Input: part model. Units: mm. Frame: model coordinates. A direction names the side the tool comes from. Give positions to 0.01 mm unless a question says otherwise; leave off trailing zeros. Order: outer loops, then holes, each group sorted by start corner. A loop starts at its lowest first (then second) coordinate and runs counter-clockwise, first axis right, second up. Notation, with made-up numbers: (-32.5, 17.5) - (-18.5, 17.5) arc R12 cw to (-18.5, 38.5) - close; hole circle Ø6 at (76, 39.25). An arc over 180 degrees is marked (long way). Answer in a Markdown table with one row per item. Add a question column.
from build123d import *

# Parameters (mm, degrees)
F1_DEPTH = 254
F2_R     = 1.98374
F3_R     = 3.69316
F4_R     = 1.35255
F5_DEPTH = 171.69384
F6_R     = 1.8288
F7_DEPTH = 1.70942
F8_R     = 0.762


with BuildPart() as f1:
    # F0 (on Top) → F1 (new body)
    with BuildSketch(Plane.XY):
        Polygon((0, -161.925), (0, 0), (-11.63066, 0), (-11.63066, -1.70942), (-1.70942, -1.70942), (-1.70942, -163.63442), (169.98442, -163.63442), (169.98442, -1.70942), (179.90566, -1.70942), (179.90566, 0), (168.275, 0), (168.275, -161.925), align=None)
    extrude(amount=F1_DEPTH)

    # F2
    f2_edges = [f1.edges().sort_by_distance(p)[0] for p in [
        (168.275, -161.925, 127),
        (0, -161.925, 127),
        (-1.70942, -1.70942, 127),
        (169.98442, -1.70942, 127),
    ]]
    fillet(f2_edges, radius=F2_R)

    # F3
    f3_edges = [f1.edges().sort_by_distance(p)[0] for p in [
        (0, 0, 127),
        (-1.70942, -163.63442, 127),
        (169.98442, -163.63442, 127),
        (168.275, 0, 127),
    ]]
    fillet(f3_edges, radius=F3_R)

    # F4 (on face) → F5 (cut, through all)
    with BuildSketch(Plane(origin=(-1.70942, 0, 0), x_dir=(0, -1, 0), z_dir=(-1, 0, 0))):
        with Locations((107.95, 3.175)):
            Circle(F4_R)
        with Locations((53.975, 3.175)):
            Circle(F4_R)
        with Locations((53.975, 250.825)):
            Circle(F4_R)
        with Locations((107.95, 250.825)):
            Circle(F4_R)
        with Locations((107.95, 127)):
            Circle(F4_R)
        with Locations((53.975, 127)):
            Circle(F4_R)
    extrude(amount=-F5_DEPTH, mode=Mode.SUBTRACT)

    # F6 (on face) → F7 (cut, through all)
    with BuildSketch(Plane(origin=(0, 0, 0), x_dir=(-1, 0, 0), z_dir=(0, 1, 0))):
        with Locations((-175.93691, 250.03125)):
            Circle(F6_R)
        with Locations((-175.93691, 127)):
            Circle(F6_R)
        with Locations((-175.93691, 3.96875)):
            Circle(F6_R)
        with Locations((7.66191, 3.96875)):
            Circle(F6_R)
        with Locations((7.66191, 127)):
            Circle(F6_R)
        with Locations((7.66191, 250.03125)):
            Circle(F6_R)
    extrude(amount=-F7_DEPTH, mode=Mode.SUBTRACT)

    # F8
    f8_edges = [f1.edges().sort_by_distance(p)[0] for p in [
        (-11.63066, -0.85471, 0),
        (-11.63066, -0.85471, 254),
        (179.90566, -0.85471, 254),
        (179.90566, -0.85471, 0),
    ]]
    fillet(f8_edges, radius=F8_R)


solid = f1.part
Q1. Section B-B, the plane z = 64. Return loops of the section in (x, y) (3 decimals), then the cut area to 3 significant figures.
Q2. Contact query for flat-ended pins moving along their axis: P1, Ø4.5, axis at y = -53.975, z = 250.825, coming from the -X side; P2, Ø3.5, axis at y = -107.95, z = 250.825, coming from the +X side; P3, Ø12, axis at x = 61, z = 36, coming from the +Y side (3 decimals). Output: stop coordinate, or through.
Q3. Pull-direction query (X, two-part tool) for faces 4 (the flat face through (169.984, -83, 125)), 5 (the flat face through (168.275, -81, 125)), 6 (the flat face through (175, 0, 125)); classes: +X half, -X half, draft (parallel to the pull), parting line (faces both ways), or undercut.
Q4. Access query for faces 1 (the flat face through (-7, -1.709, 125)), 2 (the flat face through (175, -1.709, 125)), 3 (the flat face through (85, -161.925, 125)). Directions: +Z, -Z, +X, -X, +Y, -Y. A direction counts if a zero-diameter tool reaches every point of the face in a straight line with its end or side. Return the directions, or none.
Q5. Section A-A, the plane y = -39. Return loops of the section in (x, z) (3 decimals).
Q6. Line query: probe 1 along Z at (x, y) = (-0.55, -107.95); probe 2 along X at (y, z) = (-95.5, 12) (3 decimals); probe 3 along Y at (x, z) = (168.9, 127). Output: solid intervals per line, ascending.
Q7. Section C-C, the plane x = 115. Return loops of the section in (y, z) (3 decimals).
Computed:
| question | item | result |
|---|---|---|
| 1 | outline | (-11.631, -1.709) - (-3.693, -1.709) arc R1.984 cw to (-1.709, -3.693) - (-1.709, -159.941) arc R3.693 ccw to (1.984, -163.634) - (166.291, -163.634) arc R3.693 ccw to (169.984, -159.941) - (169.984, -3.693) arc R1.984 cw to (171.968, -1.709) - (179.906, -1.709) - (179.906, 0) - (171.968, 0) arc R3.693 ccw to (168.275, -3.693) - (168.275, -159.941) arc R1.984 cw to (166.291, -161.925) - (1.984, -161.925) arc R1.984 cw to (0, -159.941) - (0, -3.693) arc R3.693 ccw to (-3.693, 0) - (-11.631, 0) - close |
| 1 | area | 873 mm^2 |
| 2 | P1 | stops at x = -1.71 |
| 2 | P2 | stops at x = 169.98 |
| 2 | P3 | stops at y = -161.925 |
| 3 | face 4 | +X half |
| 3 | face 5 | undercut |
| 3 | face 6 | draft |
| 4 | face 1 | +Z, -Z, -X, -Y |
| 4 | face 2 | +Z, -Z, +X, -Y |
| 4 | face 3 | +Z, -Z, +Y |
| 5 | outline | (-1.709, 0) - (0, 0) - (0, 254) - (-1.709, 254) - close; (168.275, 0) - (169.984, 0) - (169.984, 254) - (168.275, 254) - close |
| 6 | probe 1 | z = 0 to 1.82, 4.53 to 125.65, 128.35 to 249.47, 252.18 to 254 |
| 6 | probe 2 | x = -1.709 to 0, 168.275 to 169.984 |
| 6 | probe 3 | y = -162.56 to -109.3, -106.6 to -55.33, -52.62 to -1.64 |
| 7 | outline | (-163.634, 0) - (-161.925, 0) - (-161.925, 254) - (-163.634, 254) - close |
